Model file for the job. Use its own axes, mm. Round coordinates to 2 decimals unless told otherwise and drop trailing zeros. Use a Markdown table: item, result. Add a question column.
Item 1: Pin check, flat tips, straight feed: P1, Ø0.8, axis at y = 1, z = 0.5, coming from the +X side; P2, Ø1.5, axis at x = -40.5, z = -1, coming from the +Y side; P3, Ø2, axis at x = -88.5, z = -0.5, coming from the -Y side. Stop position of each tip, or through.
Item 2: Saw through at A-A on y = 1.5. Give the number of separate pieces and of enclosed holes in the cut face, then the cut area to 3 significant figures.
Item 3: Wall check: L1, parallel to Y at x = 82, z = -0.3. Give the ranges that are in metal, low to high. Write a range as from..to.
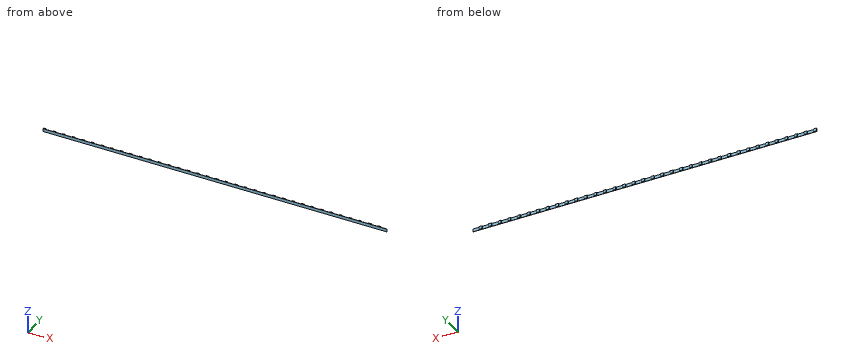
```python
from build123d import *

# Parameters (mm, degrees)
SKETCH_1_W             = 600
SKETCH_1_H             = 5
EXTRUDE_1_DEPTH        = 0.5
SKETCH_2_W             = 5
SKETCH_2_H             = 5
EXTRUDE_2_DEPTH        = 1.7
PATTERN_LINEAR_1_COUNT = 36
PATTERN_LINEAR_1_PITCH = 16.666666667


with BuildPart() as part:
    # 草图1 → 凸台-拉伸1 (new body)
    with BuildSketch(Plane(origin=(0, 0, 0), x_dir=(1, 0, 0), z_dir=(0, 1, 0))):
        Rectangle(SKETCH_1_W, SKETCH_1_H)
    extrude(amount=EXTRUDE_1_DEPTH)

    # 草图2 → 凸台-拉伸2 (add)
    with BuildSketch(Plane(origin=(0, 0.5, 0), x_dir=(1, 0, 0), z_dir=(0, 1, 0))):
        with Locations((-297.5, 0)):
            Rectangle(SKETCH_2_W, SKETCH_2_H)
    extrude_2 = extrude(amount=EXTRUDE_2_DEPTH)

    # 阵列(线性)1: 凸台-拉伸2 ×36
    with Locations(*[(i * PATTERN_LINEAR_1_PITCH, 0, 0) for i in range(1, PATTERN_LINEAR_1_COUNT)]):
        add(extrude_2)


solid = part.part
```
Entries:
| question | item | result |
|---|---|---|
| 1 | P1 | x = 288.33 |
| 1 | P2 | y = 0.5 |
| 1 | P3 | y = 0 |
| 2 | separate pieces | 36 |
| 2 | enclosed holes | 0 |
| 2 | area | 900 mm2 |
| 3 | L1 | 0..0.5 |
